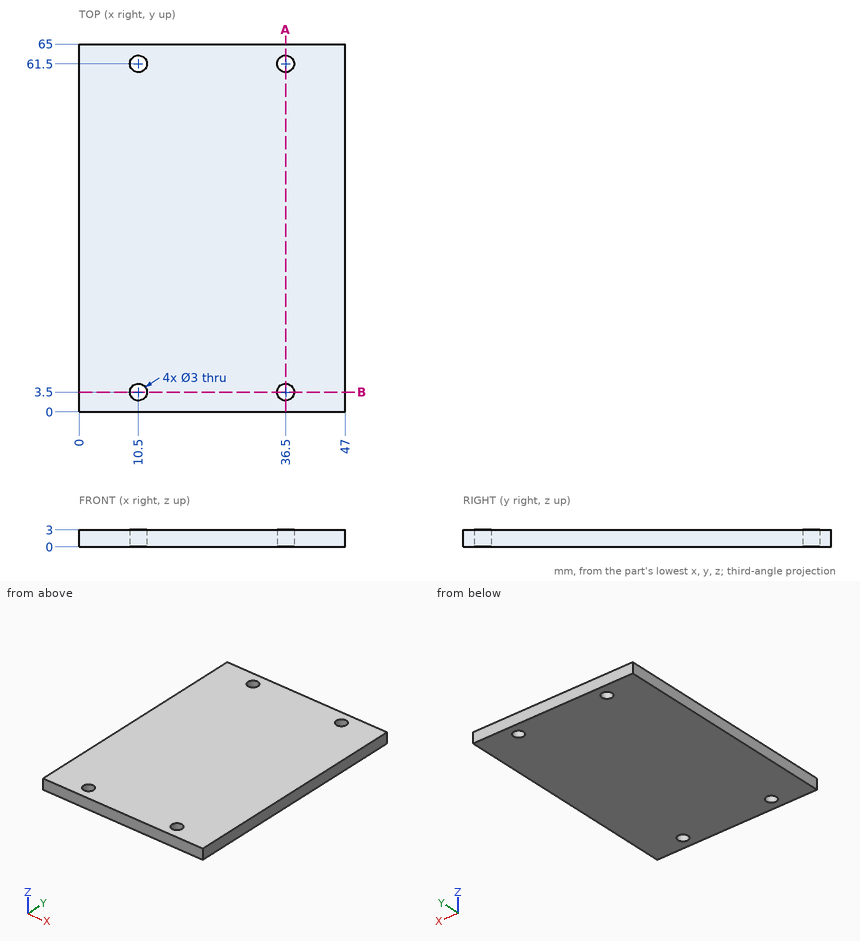
Could you check a few things on this drawing? It's one solid part, dimensions in mm from its lowest x, y, z. Give positions to 0.01 mm unless a question says otherwise; leave off trailing zeros. Write each loop counter-clockwise with the first axis right and the second up, starting at its lowest first coordinate (ties: lowest second). Pieces come first, ordered by that corner, then holes. Notation, with made-up numbers: (69, 39) -> (94, 39) arc R26 cw to (94, 66) -> close; hole circle Ø2 at (51.5, 29.25). An arc over 180 degrees is marked (long way). Answer as a JSON object with one key per item and string values.
Q1. Suppose I cut it at A-A on x = 36.5. Write out the boundary of the cut face in (y, z).
Taken from the geometry:
{"outline": "(0, 0) -> (2, 0) -> (2, 3) -> (0, 3) -> close; (5, 0) -> (60, 0) -> (60, 3) -> (5, 3) -> close; (63, 0) -> (65, 0) -> (65, 3) -> (63, 3) -> close"}
Q2. Suppose I cut it at B-B on y = 3.5. Write out the boundary of the cut face in (x, z).
Taken from the geometry:
{"outline": "(0, 0) -> (9, 0) -> (9, 3) -> (0, 3) -> close; (12, 0) -> (35, 0) -> (35, 3) -> (12, 3) -> close; (38, 0) -> (47, 0) -> (47, 3) -> (38, 3) -> close"}
Q3. Will this pin go through, and if not, where does the flat tip stop? pin 1 Ø2.5 at (x, y) = (10.5, 61.5) entering from +Z.
Taken from the geometry:
{"pin 1": "passes through"}
Q4. Please list where these lines run through material, in increasing order: L1, parallel to Y at x = 36.5, z = 1.25; L2, parallel to Y at x = 11.5, z = 1.05.
Taken from the geometry:
{"L1": "y = 0 to 2, 5 to 60, 63 to 65", "L2": "y = 0 to 2.38, 4.62 to 60.38, 62.62 to 65"}
